```python
from build123d import *

# Parameters (mm, degrees)
F0_R      = 1.5875
F1_DEPTH  = 203.2
F2_W      = 3.81
F2_H      = 4.445
F3_DEPTH  = 25.4
F5_DEPTH  = 25.4
F6_W      = 6.858
F6_H      = 6.858
F7_DEPTH  = 25.4
F6_W_2    = 6.35
F8_DEPTH  = 25.4
F9_W      = 3.175
F9_H      = 25.4
F10_DEPTH = 3.81
F11_W     = 3.175
F11_H     = 25.4
F12_DEPTH = 3.81


with BuildPart() as f1:
    # F0 (on Top) → F1 (new body)
    with BuildSketch(Plane.XY):
        Polygon((46.99, 34.29), (-59.69, 34.29), (-59.69, 8.89), (-12.7, 8.89), (-12.7, 15.24), (-38.1, 15.24), (-38.1, 27.94), (25.4, 27.94), (25.4, 15.24), (0, 15.24), (0, 8.89), (46.99, 8.89), align=None)
        with Locations((-4.7625, 31.077515)):
            Circle(F0_R, mode=Mode.SUBTRACT)
    extrude(amount=F1_DEPTH)

    # F2 (on face) → F3 (cut)
    with BuildSketch(Plane(origin=(0, 34.29, 0), x_dir=(-1, 0, 0), z_dir=(0, 1, 0))):
        with Locations((56.515, 205.4225)):
            Rectangle(F2_W, F2_H)
    extrude(amount=-F3_DEPTH, mode=Mode.SUBTRACT)

    # F4 (on face) → F5 (cut)
    with BuildSketch(Plane(origin=(0, 34.29, 0), x_dir=(-1, 0, 0), z_dir=(0, 1, 0))):
        Polygon((-41.91, 207.644923), (-45.72, 207.644923), (-45.72, 203.2), (-41.928444, 203.2), align=None)
    extrude(amount=-F5_DEPTH, mode=Mode.SUBTRACT)

    # F6 (on face) → F7 (cut)
    with BuildSketch(Plane(origin=(0, 0, 0), x_dir=(1, 0, 0), z_dir=(0, 0, -1))):
        with Locations((-49.149, -21.336)):
            Rectangle(F6_W, F6_H)
    extrude(amount=-F7_DEPTH, mode=Mode.SUBTRACT)

    # F6 (on face) → F8 (join)
    with BuildSketch(Plane(origin=(0, 0, 0), x_dir=(1, 0, 0), z_dir=(0, 0, -1))):
        with Locations((36.195, -21.336)):
            Rectangle(F6_W_2, F6_H)
    extrude(amount=F8_DEPTH)

    # F9 (on face) → F10 (cut)
    with BuildSketch(Plane(origin=(0, 0, 0), x_dir=(1, 0, 0), z_dir=(0, 0, -1))):
        with Locations((-56.8325, -21.59)):
            Rectangle(F9_W, F9_H)
    extrude(amount=-F10_DEPTH, mode=Mode.SUBTRACT)

    # F11 (on face) → F12 (cut)
    with BuildSketch(Plane(origin=(0, 0, 0), x_dir=(1, 0, 0), z_dir=(0, 0, -1))):
        with Locations((44.1325, -21.59)):
            Rectangle(F11_W, F11_H)
    extrude(amount=-F12_DEPTH, mode=Mode.SUBTRACT)


solid = f1.part
```
Here's how the part is built. I have some questions about the finished solid (model axes, mm). A direction names the side the tool comes from. Give positions to 0.01 mm unless a question says otherwise; leave off trailing zeros. Loops run counter-clockwise (first coordinate to the right, second up) from the corner with the lowest first, then second, coordinate; pieces in that order, holes last. Notation, with made-up numbers: (12.5, 53) -> (25.5, 53) arc R16 cw to (25.5, 73) -> close; hole circle Ø8 at (46.25, 27.5). An arc over 180 degrees is marked (long way). Use one line per item in the form item = value. Start each with the question number.
1) Which directions (+Z, -Z, +X, -X, +Y, -Y) give clear straight access to the entire face, cutting with the end or side of a thin tool? Please do faces 4 (the face through (-55.245, 22, 2)), 5 (the face through (-38.1, 22, 100)), 6 (the face through (0, 12, 100)), 7 (the face through (-52.578, 21, 13)).
2) Imagine slicing it at C-C (z = 131). Please give me the cut outline in (x, y) (1 decimal).
3) Thinking about a two-plate mould opening in Y: for faces 1 (the face through (36, 24.765, -13)), 2 (the face through (13, 15.24, 100)), 3 (the face through (45.72, 22, 2)), which applies, +Y half, -Y half, draft (parallel to the pull), parting line (faces both ways), or undercut?
4) Imagine slicing it at B-B (y = 22). Please give me the cut outline in (x, z) (3 decimals), then the cut area to 3 significant figures.
5) Please list where these lines run through material, in increasing order: line 1 along X through (y, z) = (27.25, 2) (3 decimals); line 2 along X through (y, z) = (23.25, 85.5); line 3 along X through (y, z) = (14.25, 108).
6) For P1, Ø1.4, axis at x = 46.5, y = 27, coming from the -Z side; P2, Ø5.5, axis at y = 22.5, z = -12, coming from the +X side, each with a flat end and sliding along its axis, tell me the tip position at first contact or that it passes through.
7) Imagine slicing it at D-D (z = 23). Please give me the cut outline in (x, y) (1 decimal), then the cut area to 3 significant figures.
8) Imagine slicing it at A-A (x = -25). Please give me the cut outline in (y, z).
Check values:
q1.face_4 = -Z, +Y, -Y
q1.face_5 = +Z, -Z
q1.face_6 = +Z, -Z, -Y
q1.face_7 = -Z
q2.outline = (-59.7, 8.9) -> (-12.7, 8.9) -> (-12.7, 15.2) -> (-38.1, 15.2) -> (-38.1, 27.9) -> (25.4, 27.9) -> (25.4, 15.2) -> (0, 15.2) -> (0, 8.9) -> (47, 8.9) -> (47, 34.3) -> (-59.7, 34.3) -> close; hole circle Ø3.2 at (-4.8, 31.1)
q3.face_1 = +Y half
q3.face_2 = undercut
q3.face_3 = draft
q4.outline = (-59.69, 0) -> (-58.42, 0) -> (-58.42, 3.81) -> (-55.245, 3.81) -> (-55.245, 0) -> (-52.578, 0) -> (-52.578, 25.4) -> (-45.72, 25.4) -> (-45.72, 0) -> (-38.1, 0) -> (-38.1, 203.2) -> (-59.69, 203.2) -> close; (25.4, 0) -> (33.02, 0) -> (33.02, -25.4) -> (39.37, -25.4) -> (39.37, 0) -> (42.545, 0) -> (42.545, 3.81) -> (45.72, 3.81) -> (45.72, 0) -> (46.99, 0) -> (46.99, 203.2) -> (25.4, 203.2) -> close
q4.area = 8,740 mm^2
q5.line_1 = -59.69 to -58.42, -55.245 to -38.1, 25.4 to 42.545, 45.72 to 46.99
q5.line_2 = -59.69 to -38.1, 25.4 to 46.99
q5.line_3 = -59.69 to -12.7, 0 to 46.99
q6.P1 = 0
q6.P2 = 39.37
q7.outline = (-59.7, 8.9) -> (-12.7, 8.9) -> (-12.7, 15.2) -> (-38.1, 15.2) -> (-38.1, 27.9) -> (25.4, 27.9) -> (25.4, 15.2) -> (0, 15.2) -> (0, 8.9) -> (47, 8.9) -> (47, 34.3) -> (-59.7, 34.3) -> close; hole (-52.6, 17.9) -> (-45.7, 17.9) -> (-45.7, 24.8) -> (-52.6, 24.8) -> close; hole circle Ø3.2 at (-4.8, 31.1)
q7.area = 1,770 mm^2
q8.outline = (8.89, 0) -> (15.24, 0) -> (15.24, 203.2) -> (8.89, 203.2) -> close; (27.94, 0) -> (34.29, 0) -> (34.29, 203.2) -> (27.94, 203.2) -> close
